Work out the finished part from the listing and answer in its coordinate system (mm). A direction names the side the tool comes from. Coordinates: 2 decimals unless noted, no trailing zeros. Loops run counter-clockwise (first coordinate to the right, second up) from the corner with the lowest first, then second, coordinate; pieces in that order, holes last. Notation, with made-up numbers: (2, 89.5) - (22, 89.5) arc R35 ccw to (22, 124.5) - close; hole circle Ø3 at (-21.5, 21.25). An arc over 180 degrees is marked (long way). Write each question's results on one line, items separated by ' | '. Start each with the question number.
1. Each of these flat-tipped pins is pushed along its axis until it touches: P1, Ø10, axis at x = -6.5, y = 44, coming from the -Z side; P2, Ø11, axis at y = 35, z = 0, coming from the +X side; P3, Ø3.5, axis at x = 10, z = -10, coming from the +Y side. Where does it stop, or does it pass through?
2. Which of the six approach directions +Z, -Z, +X, -X, +Y, -Y give full straight-line access (tool end or side, diameter ignored) to faces 4 (the cylindrical face through (9.909, 7.605, -7.935)), 5 (the flat face through (-0.21, 44.08, -11.49))?
3. Determine the mould class of faces 1 (the flat face through (15, 25, 0)), 2 (the conical face through (-10.31, 15.99, -10.16)), 3 (the cylindrical face through (10.44, 33.78, 10.16)) for opening direction Y: released by +Y, released by -Y, zero draft, split by the parting line, or undercut.
4. A cutting plane is placed at C-C on y = 32.5. Determine the outline of the cut face in (x, z), then the cut area to 3 significant figures.
5. A cutting plane is placed at B-B on y = 9.5. Determine the outline of the cut face in (x, z).
6. A cutting plane is placed at A-A on z = 0. Determine the outline of the cut face in (x, y).
7. Find the intervals of material crossed by line 1 along Z through (x, y) = (10, 10); line 2 along X through (y, z) = (5.75, -10), in increasing order. Write a range as [from, to].
Autodesk Inventor part; units mm, degrees
ref_plane "Work Plane1" through (6.35, 0, 0) normal (1, 0, 0) x (0, 1, 0)
ref_plane "XZ Plane" through (0, 0, 0) normal (0, 1, 0) x (-1, 0, 0)
ref_plane "XY Plane" through (0, 0, 0) normal (0, 0, 1) x (1, 0, 0)
sketch "Sketch1" plane through (0, 0, 0) normal (0, 1, 0) x (-1, 0, 0)
  line L0 (-15, -15) -> (15, -15)
  line L1 (15, -15) -> (15, 15)
  line L2 (15, 15) -> (-15, 15)
  line L3 (-15, 15) -> (-15, -15)
  line L4 (-15, -15) -> (15, 15) construction
  line L5 (15, -15) -> (-15, 15) construction
  point P0 (0, 0)
  dimension "d0" = 30
  dimension "d1" = 30
extrude "Extrusion1" add sketch "Sketch1" along normal blind 50
sketch "Sketch2" plane through (15, 0, 15) normal (1, 0, 0) x (0, 0, -1)
  line L0 (15, 0) -> (15, 35) construction
  line L1 (0, 0) -> (30, 0)
  circle A0 centre (15, 35) radius 6
  dimension "d4" = 35
  dimension "d6" = 12
extrude "Extrusion2" cut sketch "Sketch2" against normal through all
sketch "Sketch7" plane through (0, 50, 0) normal (0, 1, 0) x (1, 0, 0)
  line L0 (15, -15) -> (15, 15)
  line L1 (6.5, 0) -> (6.35, 0)
  circle A0 centre (6.35, 0) radius 2.25
  point P0 (0, 0)
  dimension "d33" = 4.5
  dimension "d119" = 8.65
extrude "Extrusion7" cut sketch "Sketch7" against normal blind 12
ref_plane "Work Plane1" through (6.35, 0, 0) normal (1, 0, 0) x (0, 1, 0)
sketch "Sketch14" plane through (6.35, 0, 0) normal (1, 0, 0) x (0, 1, 0)
  line L0 (50, -15) -> (50, 15)
  circle A0 centre (35, 0) radius 6
  line L1 (50, 0) -> (35, 0)
  line L2 (35, 0) -> (52.3205, -30)
  line L3 (35, 0) -> (61.673, 0)
  line L4 (35, 0) -> (36.7321, 0)
  line L5 (36.7321, 0) -> (54.0526, -30)
  line L6 (54.0526, -30) -> (52.3205, -30)
  line L7 (52, -6.9171) -> (34.5359, -17)
  line L8 (34.5359, -17) -> (52, -17)
  line L9 (52, -17) -> (52, -6.9171)
  line L10 (0, -15) -> (50, -15)
  line L11 (0, -15) -> (50, -15)
  point P0 (0, 0)
  point P1 (36.7321, 0)
  point P2 (38, -15)
  dimension "d55" = 60
  dimension "d57" = 120
  dimension "d72" = 1.5
  dimension "d73" = 30
  dimension "d112" = 2
  dimension "d113" = 2
  dimension "d114" = 12
revolve "Revolution1" cut sketch "Sketch14" angle 360 about axis through (6.35, 35, 0) along (0, 0.5, -0.8660254) contours L10 L2 L7 L5 | L5 L8 L2 L10 | L7 L2 A0 L5 | L5 L6 L2 L8 | A0 L2 L1 L5
extrude "Extrusion11" cut sketch "Sketch14" along normal blind 99 and the other way blind 99 contours L10 L5 L7 L0 | L0 L7 L9 L8 L5 L10 | L10 L2 L7 L5 | L5 L8 L2 L10 | L10 L7 L2 | L2 L8 L7 L10
mirror "Mirror4" about plane through (0, 0, 0) normal (0, 0, 1) of "Revolution1", "Extrusion11"
sketch "Sketch19" plane through (0, 0, 0) normal (0, -1, 0) x (1, 0, 0)
  point P0 (0, 0)
  point P1 (-10, 10)
  point P2 (10, -10)
  dimension "d97" = 10
  dimension "d98" = 10
  dimension "d99" = 10
  dimension "d100" = 10
hole "Hole2" at (-10, 0, 10) at (10, 0, -10) direction (0, 1, 0) diameter 4.134 depth 15 tip angle 118
sketch "Sketch20" plane through (0, 0, 0) normal (0, -1, 0) x (1, 0, 0)
  point P0 (0, 0)
  point P1 (10, 10)
  point P2 (-10, -10)
  dimension "d108" = 10
  dimension "d109" = 10
  dimension "d110" = 10
  dimension "d111" = 10
hole "Hole3" at (10, 0, 10) at (-10, 0, -10) direction (0, 1, 0) diameter 4 depth 15 tip angle 118
sketch "Sketch21" plane through (15, 0, 15) normal (1, 0, 0) x (0, 0, -1)
  line L0 (0, 0) -> (30, 0)
  circle A0 centre (15, 35) radius 6
  point P0 (15, 0)
  point P1 (5, 35)
  point P2 (25, 35)
  point P3 (15, 0)
  point P4 (15, 0)
  dimension "d127" = 10
  dimension "d128" = 10
hole "Hole4" at (15, 35, 10) at (15, 35, -10) direction (-1, 0, 0) diameter 2.459 depth 9 tip angle 118
properties part number "23-0064 Diode holder" material "Stainless Steel 316 (X5CrNiMo17.12.2)"
Values:
1) P1: z = -14.42 | P2: through | P3: y = 49.69
2) face 4: -Y | face 5: -Z, +X, -X, +Y
3) face 1: zero draft | face 2: released by -Y | face 3: undercut
4) outline: (-15, -15) - (15, -15) - (15, -5.45) - (-15, -5.45) - close; (-15, 5.45) - (15, 5.45) - (15, 15) - (-15, 15) - close | area: 573 mm^2
5) outline: (-15, -15) - (15, -15) - (15, 15) - (-15, 15) - close; hole circle Ø4.13 at (-10, 10); hole circle Ø4 at (-10, -10); hole circle Ø4.13 at (10, -10); hole circle Ø4 at (10, 10)
6) outline: (-15, 0) - (15, 0) - (15, 29) - (-15, 29) - close; (-15, 41) - (4.1, 41) - (4.1, 50) - (-15, 50) - close; (8.6, 41) - (15, 41) - (15, 50) - (8.6, 50) - close
7) line 1: [-15, -12.07], [-7.93, 8], [12, 15] | line 2: [-15, -12], [-8, 7.93], [12.07, 15]
